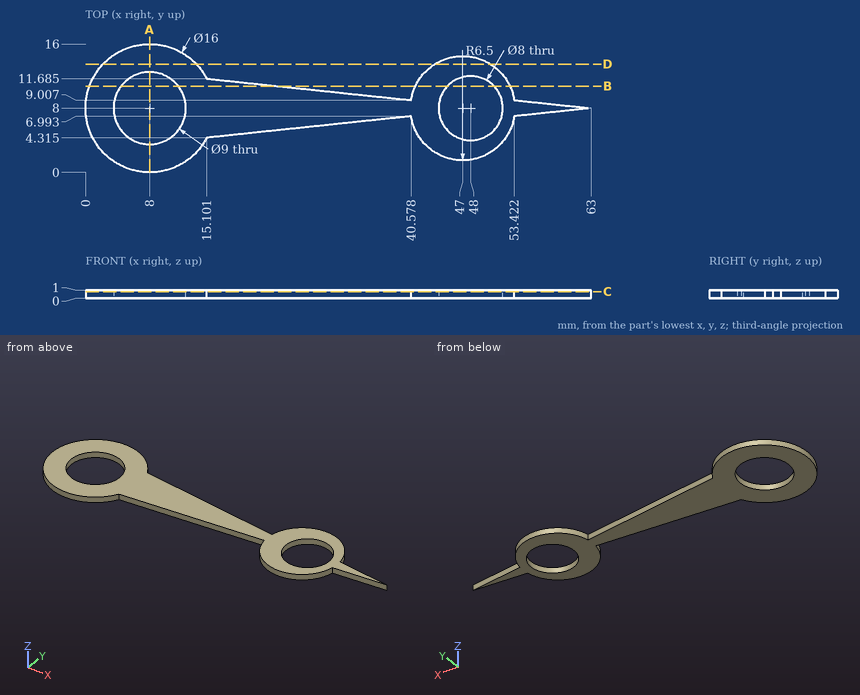
Part print with two shaded views. Sizes in mm from the minimum x, y, z corner. Coordinates: 2 decimals unless noted, no trailing zeros. Write each loop counter-clockwise with the first axis right and the second up, starting at its lowest first coordinate (ties: lowest second). Pieces come first, ordered by that corner, then holes.
(1) Cut at C-C on z = 0.85. List the corners of the cut face in (x, y) (1 decimal).
(2) Cut at B-B on y = 10.75. List the corners of the cut face in (x, z) (1 decimal).
(3) Pin check, flat tip, straight feed: pin 1 Ø5.5 at (x, y) = (8, 8) entering from -Z. Stop position of the tip, or through.
(4) Cut at A-A on x = 8. List the corners of the cut face in (y, z).
(5) Drill centre lines: line 1 (Y direction, x = 8, z = 0.5); line 2 (Y direction, x = 6, z = 0.55) (1 decimal); line 3 (Y direction, x = 53, z = 0.35) (1 decimal). Where is each one in solid material? Low to high.
(6) Cut at D-D on y = 13.5. List the corners of the cut face in (x, z) (1 decimal).
Working result:
1. outline: (15.1, 4.3) - (40.6, 7) arc R6.5 ccw to (53.4, 7) - (63, 8) - (53.4, 9) arc R6.5 ccw to (40.6, 9) - (15.1, 11.7) arc R8 ccw (long way) to start; hole circle Ø9 at (8, 8); hole circle Ø8 at (48, 8)
2. outline: (0.5, 0) - (4.4, 0) - (4.4, 1) - (0.5, 1) - close; (11.6, 0) - (24, 0) - (24, 1) - (11.6, 1) - close; (41.1, 0) - (45.1, 0) - (45.1, 1) - (41.1, 1) - close; (50.9, 0) - (52.9, 0) - (52.9, 1) - (50.9, 1) - close
3. pin 1: passes through
4. outline: (0, 0) - (3.5, 0) - (3.5, 1) - (0, 1) - close; (12.5, 0) - (16, 0) - (16, 1) - (12.5, 1) - close
5. line 1: y = 0 to 3.5, 12.5 to 16
5. line 2: y = 0.3 to 4, 12 to 15.7
5. line 3: y = 5.5 to 10.5
6. outline: (2.2, 0) - (13.8, 0) - (13.8, 1) - (2.2, 1) - close; (43.5, 0) - (50.5, 0) - (50.5, 1) - (43.5, 1) - close
